```python
from build123d import *

# Parameters (mm, degrees)
SKETCH1_W                       = 25
SKETCH1_H                       = 25
BOSS_EXTRUDE1_DEPTH             = 15
SKETCH2_W                       = 19
SKETCH2_H                       = 14
CUT_EXTRUDE1_DEPTH              = 5
CUT_EXTRUDE2_DEPTH              = 24.184046239
CUT_EXTRUDE2_DEPTH_BACK         = 15
SKETCH3_W                       = 19
SKETCH3_H                       = 5.5
TAP_DRILL_FOR_M3X0_5_TAP1_D     = 2.5
TAP_DRILL_FOR_M3X0_5_TAP1_DEPTH = 5
TAP_DRILL_FOR_M3X0_5_TAP1_TIP   = 0.751075774
SKETCH6_W                       = 2
SKETCH6_H                       = 2
BOSS_EXTRUDE2_DEPTH             = 25
SKETCH7_W                       = 1
SKETCH7_H                       = 1
BOSS_EXTRUDE3_DEPTH             = 25


with BuildPart() as part:
    # Sketch1 → Boss-Extrude1 (new body)
    with BuildSketch(Plane(origin=(0, 0, 0), x_dir=(1, 0, 0), z_dir=(0, 1, 0))):
        Rectangle(SKETCH1_W, SKETCH1_H)
    extrude(amount=BOSS_EXTRUDE1_DEPTH)

    # Sketch2 → Cut-Extrude1 (cut)
    with BuildSketch(Plane(origin=(0, 15, 0), x_dir=(1, 0, 0), z_dir=(0, 1, 0))):
        Rectangle(SKETCH2_W, SKETCH2_H)
    extrude(amount=-CUT_EXTRUDE1_DEPTH, mode=Mode.SUBTRACT)

    # Sketch3 → Cut-Extrude2 (cut, two sides: drawn at the far end of the back side and taken through both)
    with BuildSketch(Plane(origin=(0, 15, 0), x_dir=(1, 0, 0), z_dir=(0, 1, 0)).offset(-CUT_EXTRUDE2_DEPTH_BACK)):
        with Locations((0, -9.75)):
            Rectangle(SKETCH3_W, SKETCH3_H)
    extrude(amount=CUT_EXTRUDE2_DEPTH + CUT_EXTRUDE2_DEPTH_BACK, mode=Mode.SUBTRACT)

    # Tap Drill for M3x0.5 Tap1
    with Locations(Plane(origin=(-7.5, 15, -9.75), x_dir=(0, 0, 1), z_dir=(0, 1, 0))):
        with Locations((0, 0), (0, 15)):
            Hole(TAP_DRILL_FOR_M3X0_5_TAP1_D / 2, depth=TAP_DRILL_FOR_M3X0_5_TAP1_DEPTH)
            with Locations((0, 0, -(TAP_DRILL_FOR_M3X0_5_TAP1_DEPTH + TAP_DRILL_FOR_M3X0_5_TAP1_TIP / 2))):  # 118° drill point
                Cone(0, TAP_DRILL_FOR_M3X0_5_TAP1_D / 2, TAP_DRILL_FOR_M3X0_5_TAP1_TIP, mode=Mode.SUBTRACT)

    # Sketch6 → Boss-Extrude2 (add)
    with BuildSketch(Plane(origin=(12.5, 0, 0), x_dir=(0, 0, -1), z_dir=(1, 0, 0))):
        with Locations((13.5, 3.5)):
            Rectangle(SKETCH6_W, SKETCH6_H)
    extrude(amount=-BOSS_EXTRUDE2_DEPTH)

    # Sketch7 → Boss-Extrude3 (add)
    with BuildSketch(Plane(origin=(12.5, 0, 0), x_dir=(0, 0, -1), z_dir=(1, 0, 0))):
        with Locations((14, 5)):
            Rectangle(SKETCH7_W, SKETCH7_H)
    extrude(amount=-BOSS_EXTRUDE3_DEPTH)


solid = part.part
```
Input: part model. Units: mm. Frame: model coordinates. A direction names the side the tool comes from. Give positions to 0.01 mm unless a question says otherwise; leave off trailing zeros. Write each loop counter-clockwise with the first axis right and the second up, starting at its lowest first coordinate (ties: lowest second). Pieces come first, ordered by that corner, then holes. Notation, with made-up numbers: (-26, 64) - (27, 64) arc R29 ccw to (27, 84) - close; hole circle Ø1 at (87.25, 2). An arc over 180 degrees is marked (long way). Write item = value, one per line. Start each with the question number.
1. Ray query, L1, parallel to X at y = 11.35, z = -9.75; L2, parallel to X at y = 13, z = 5.5; L3, parallel to Z at x = -7.5, y = 11.35. Return the intervals inside material, ascending.
2. Mould query, pull axis X, two halves, no side actions, for faces 1 (the flat face through (9.5, 11, 5)), 2 (the flat face through (0, 5.5, -14)), 3 (the flat face through (-12.5, 8, -1)). Classes: released by +X, released by -X, zero draft, split by the parting line, or undercut.
3. Section query B-B, the plane y = 7. Output: boundary loops of the cut face in (x, z), then the cut area to 4 significant figures.
4. First-contact query: pin 1 Ø0.5 at (x, z) = (-2.5, -13) entering from +Y; pin 2 Ø2 at (x, z) = (5.5, -3) entering from +Y; pin 3 Ø1.5 at (x, z) = (7.5, -9.75) entering from -Y; pin 4 Ø0.8 at (x, y) = (-4.5, 1.5) entering from -Z. Flat tips, straight axial feed; report the tip coordinate or a pass-through.
5. Access query for faces 4 (the cylindrical face through (-7.45, 12.46, -8.5)), 5 (the flat face through (0, 13, -7)), 6 (the flat face through (0, 4.5, -13)), 7 (the flat face through (0, 2.5, -13)). Directions: +Z, -Z, +X, -X, +Y, -Y. A direction counts if a zero-diameter tool reaches every point of the face in a straight line with its end or side. Return the directions, or none.
6. Section query C-C, the plane x = -2. Output: boundary loops of the cut face in (y, z), then the cut area to 4 significant figures.
7. Section query A-A, the plane y = 10.5. Output: boundary loops of the cut face in (x, z), then the cut area to 3 significant figures.
8. Section query D-D, the plane z = -6. Output: boundary loops of the cut face in (x, y), then the cut area to 3 significant figures.
Check sheet entries:
q1.L1 = -12.5 to -8.75, -6.25 to 6.25, 8.75 to 12.5
q1.L2 = -12.5 to -9.5, 9.5 to 12.5
q1.L3 = -12.5 to -11, -8.5 to -7
q2.face_1 = undercut
q2.face_2 = zero draft
q2.face_3 = released by -X
q3.outline = (-12.5, -12.5) - (12.5, -12.5) - (12.5, 12.5) - (9.5, 12.5) - (9.5, 7) - (-9.5, 7) - (-9.5, 12.5) - (-12.5, 12.5) - close
q3.area = 520.5 mm2
q4.pin_1 = 4.5
q4.pin_2 = 10
q4.pin_3 = 0
q4.pin_4 = -12.5
q5.face_4 = +Y
q5.face_5 = +Z, +Y
q5.face_6 = +X, -X, +Y
q5.face_7 = -Z, +X, -X, -Y
q6.outline = (0, -12.5) - (2.5, -12.5) - (2.5, -14.5) - (5.5, -14.5) - (5.5, -13.5) - (4.5, -13.5) - (4.5, -12.5) - (15, -12.5) - (15, -7) - (10, -7) - (10, 7) - (0, 7) - close
q6.area = 227.5 mm2
q7.outline = (-12.5, -12.5) - (12.5, -12.5) - (12.5, 12.5) - (9.5, 12.5) - (9.5, -7) - (-9.5, -7) - (-9.5, 12.5) - (-12.5, 12.5) - close; hole circle Ø2.5 at (-7.5, -9.75); hole circle Ø2.5 at (7.5, -9.75)
q7.area = 245 mm2
q8.outline = (-12.5, 0) - (12.5, 0) - (12.5, 15) - (9.5, 15) - (9.5, 10) - (-9.5, 10) - (-9.5, 15) - (-12.5, 15) - close
q8.area = 280 mm2
